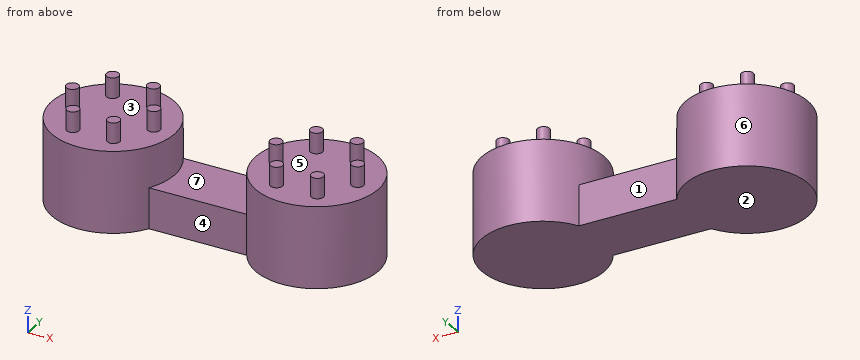
```python
from build123d import *

# Parameters (mm, degrees)
SKETCH1_R             = 15
BOSS_EXTRUDE1_DEPTH   = 20
BOSS_EXTRUDE1_2_DEPTH = 20
SKETCH2_R             = 1.5
BOSS_EXTRUDE2_DEPTH   = 5
SKETCH3_W             = 50
SKETCH3_H             = 15
BOSS_EXTRUDE3_DEPTH   = 10


with BuildPart() as part:
    # Sketch1 → Boss-Extrude1 (new body)
    with BuildSketch(Plane.XY):
        with Locations((25, 0)):
            Circle(SKETCH1_R)
    extrude(amount=BOSS_EXTRUDE1_DEPTH)



with BuildPart() as body_2:
    # Sketch1 → Boss-Extrude1 2 (new body)
    with BuildSketch(Plane.XY):
        with Locations((-25, 0)):
            Circle(SKETCH1_R)
    extrude(amount=BOSS_EXTRUDE1_2_DEPTH)


with BuildPart() as part_1:
    add(part.part)

    add(body_2.part)  # Boss-Extrude2 merges body 2
    # Sketch2 → Boss-Extrude2 (add)
    with BuildSketch(Plane.XY.offset(20)):
        with Locations((35, 0)):
            Circle(SKETCH2_R)
        with Locations((30, -8.660254038)):
            Circle(SKETCH2_R)
        with Locations((20, -8.660254038)):
            Circle(SKETCH2_R)
        with Locations((15, 0)):
            Circle(SKETCH2_R)
        with Locations((20, 8.660254038)):
            Circle(SKETCH2_R)
        with Locations((30, 8.660254038)):
            Circle(SKETCH2_R)
        with Locations((-15, 0)):
            Circle(SKETCH2_R)
        with Locations((-20, -8.660254038)):
            Circle(SKETCH2_R)
        with Locations((-30, -8.660254038)):
            Circle(SKETCH2_R)
        with Locations((-35, 0)):
            Circle(SKETCH2_R)
        with Locations((-30, 8.660254038)):
            Circle(SKETCH2_R)
        with Locations((-20, 8.660254038)):
            Circle(SKETCH2_R)
    extrude(amount=BOSS_EXTRUDE2_DEPTH)

    # Sketch3 → Boss-Extrude3 (add)
    with BuildSketch(Plane.XY):
        Rectangle(SKETCH3_W, SKETCH3_H)
    extrude(amount=BOSS_EXTRUDE3_DEPTH)


solid = part_1.part
```
The listing builds one solid part. Answer for the finished solid, in the listing's coordinates (mm). Face numbers are marked on the shaded views. A direction names the side the tool comes from. Give positions to 0.01 mm unless a question says otherwise; leave off trailing zeros. Order: outer loops, then holes, each group sorted by start corner. A loop starts at its lowest first (then second) coordinate and runs counter-clockwise, first axis right, second up. Notation, with made-up numbers: (-10.75, -4) - (1.25, -4) arc R36 cw to (1.25, 35) - close; hole circle Ø7 at (69.25, -12.75). An arc over 180 degrees is marked (long way). Answer in a Markdown table with one row per item. Add a question column.
Q1. The part is cut by section A-A (z = 22.25). Give the number of separate pieces and of enclosed holes in the cut face, then the cut area to 3 significant figures.
Q2. The part is cut by section C-C (x = 25). Determine the outline of the cut face in (y, z).
Q3. For a pull along Y with two mould halves and no side action, classify the marked faces 4, 5, 6 and 7 as released by +Y, released by -Y, zero draft, split by the parting line, or undercut.
Q4. The part is cut by section B-B (z = 17.75). Determine the outline of the cut face in (x, y), then the cut area to 3 significant figures.
Q5. The part is cut by section D-D (z = 3). Determine the outline of the cut face in (x, y), then the cut area to 3 significant figures.
Q6. Find the intervals of material crossed by line 1 along X through (y, z) = (-0.25, 5.5); line 2 along Y through (x, z) = (24.5, 12.25); line 3 along Z through (x, y) = (-14, -8.75), in increasing order. Write a range as [from, to].
Q7. Which of the six approach directions +Z, -Z, +X, -X, +Y, -Y give full straight-line access (tool end or side, diameter ignored) to the marked faces 1, 2 and 3?
Q8. Given P1, Ø4, axis at y = -4.5, z = 6.5, coming from the -X side; P2, Ø4, axis at y = 7, z = 17, coming from the +X side; P3, Ø1.5, axis at x = 25.5, y = 6, coming from the +Z side, each flat-ended and moving along its own axis, determine where each tip first touches the part or whether it passes through.
Determined:
| question | item | result |
|---|---|---|
| 1 | separate pieces | 12 |
| 1 | enclosed holes | 0 |
| 1 | area | 84.8 mm² |
| 2 | outline | (-15, 0) - (15, 0) - (15, 20) - (-15, 20) - close |
| 3 | face 4 | released by -Y |
| 3 | face 5 | undercut |
| 3 | face 6 | split by the parting line |
| 3 | face 7 | zero draft |
| 4 | outline | circle Ø30 at (-25, 0); circle Ø30 at (25, 0) |
| 4 | area | 1,410 mm² |
| 5 | outline | (-12.01, -7.5) - (12.01, -7.5) arc R15 ccw (long way) to (12.01, 7.5) - (-12.01, 7.5) arc R15 ccw (long way) to start |
| 5 | area | 1,730 mm² |
| 6 | line 1 | x = [-40, 40] |
| 6 | line 2 | y = [-14.99, 14.99] |
| 6 | line 3 | z = [0, 20] |
| 7 | face 1 | +Z, -Z, +Y |
| 7 | face 2 | -Z, +X, -X, +Y, -Y |
| 7 | face 3 | +Z |
| 8 | P1 | stops at x = -39.79 |
| 8 | P2 | stops at x = 39.14 |
| 8 | P3 | stops at z = 20 |
